Input: part model. Units: mm. Frame: model coordinates. Face numbers are marked on the shaded views. A direction names the side the tool comes from. Round coordinates to 2 decimals unless told otherwise and drop trailing zeros. Write each loop counter-clockwise with the first axis right and the second up, starting at its lowest first coordinate (ties: lowest second). Pieces come first, ordered by that corner, then holes. Notation, with made-up numbers: (9.25, -28.5) -> (34.25, -28.5) arc R8 ccw to (34.25, -19.5) -> close; hole circle Ø10 at (57.25, -26). An arc over 180 degrees is marked (long way). Use CSV: the item, a comma, the result in double quotes.
Autodesk Fusion 360 part; units mm, degrees
sketch "Sketch1" plane through (0, 0, 0) normal (0, 1, 0) x (1, 0, 0)
  line L0 (-7, -13) -> (7, -13)
  line L1 (7, -13) -> (7, 0)
  line L2 (7, 0) -> (-7, 0)
  line L3 (-7, 0) -> (-7, -13)
  line L4 (-3.5, -13) -> (3.5, -13) construction
  line L5 (3.5, -13) -> (3.5, -8.75) construction
  line L6 (3.5, -8.75) -> (-3.5, -8.75) construction
  line L7 (-3.5, -8.75) -> (-3.5, -13) construction
  line L8 (-3.5, -11.75) -> (-2.25, -13) construction
  line L9 (2.25, -13) -> (3.5, -11.75) construction
  line L10 (0, -8.75) -> (0, 0) construction
  dimension "d3" = 7
  dimension "d4" = 1.25
  dimension "d5" = 1.25
  dimension "d6" = 3
  dimension "d7" = 45
  dimension "d8" = 3.5
  dimension "d9" = 3.5
  dimension "d10" = 13
extrude "Extrude1" add sketch "Sketch1" along normal mid plane 80
sketch "Sketch2" plane through (0, 0, 0) normal (0, 0, 1) x (1, 0, 0)
  line L0 (-7, -40) -> (7, -40)
  line L1 (7, -40) -> (7, -45)
  line L2 (2, -50) -> (-2, -50)
  line L3 (-7, -45) -> (-7, -40)
  arc A0 (2, -50) -> (7, -45) centre (2, -45) ccw
  arc A1 (-7, -45) -> (-2, -50) centre (-2, -45) ccw
  line L4 (7, -40) -> (-7, -40)
  point P0 (7, -50)
  dimension "d13" = 10
  dimension "d14" = 5
extrude "Extrude2" add sketch "Sketch2" along normal blind 5
sketch "Sketch3" plane through (0, 0, 5) normal (0, 0, 1) x (-1, 0, 0)
  line L0 (7, 40) -> (7, 45)
  arc A0 (7, 45) -> (2, 50) centre (2, 45) ccw
  line L1 (2, 50) -> (-2, 50)
  arc A1 (-2, 50) -> (-7, 45) centre (-2, 45) ccw
  line L2 (-7, 45) -> (-7, 40)
  line L3 (-7, 40) -> (7, 40)
  circle A2 centre (0, 45) radius 1.75
  line L4 (-7, 45) -> (7, 45) construction
  dimension "d20" = 3.5
extrude "Extrude3" cut sketch "Sketch3" against normal blind 5 contours A2
chamfer "Chamfer1" distance 1.5 angle 60 1 edges at (1.6316, -45.6328, 5) measured on face at (-5.1922, -43.0802, 5)
mirror "Mirror1" about plane through (0, 0, 0) normal (0, 1, 0) of "Extrude2", "Extrude3", "Chamfer1"
sketch "Sketch4" plane through (0, -40, 0) normal (0, -1, 0) x (1, 0, 0)
  line L0 (-7, 5) -> (7, 5)
  line L1 (7, 5) -> (7, 13)
  line L2 (7, 13) -> (-7, 13)
  line L3 (-7, 13) -> (-7, 5)
  line L4 (-3.5, 8.75) -> (-3.5, 13) construction
  line L5 (-3.5, 11.75) -> (-2.25, 13) construction
  line L6 (2.25, 13) -> (3.5, 11.75) construction
  line L7 (3.5, 13) -> (3.5, 8.75) construction
  line L8 (3.5, 8.75) -> (-3.5, 8.75) construction
  line L9 (3.6, 13) -> (3.6, 8.65)
  line L10 (3.6, 8.65) -> (-3.6, 8.65)
  line L11 (-3.6, 8.65) -> (-3.6, 13)
  line L12 (-2.25, 13) -> (-3.6, 11.65)
  line L13 (2.25, 13) -> (3.6, 11.65)
  dimension "d25" = -0.1
extrude "Extrude4" cut sketch "Sketch4" against normal up to surface (80 mm away) contours L2 L9 L10 L11 L12 L13
sketch "Sketch5" plane through (-7, 0, 0) normal (-1, 0, 0) x (0, -1, 0)
  line L0 (40, 13) -> (-40, 13)
  line L1 (-40, 13) -> (-40, 5)
  line L2 (-40, 5) -> (-45, 5)
  line L3 (-45, 5) -> (-45, 0)
  line L4 (-45, 0) -> (45, 0)
  line L5 (45, 0) -> (45, 5)
  line L6 (45, 5) -> (40, 5)
  line L7 (40, 5) -> (40, 13)
  line L8 (-17.5, 13) -> (17.5, 13)
  line L9 (17.5, 13) -> (17.5, 5)
  line L10 (17.5, 5) -> (-17.5, 5)
  line L11 (-17.5, 5) -> (-17.5, 13)
  line L12 (0, 0) -> (0, 5) construction
  dimension "d28" = 35
extrude "Extrude5" cut sketch "Sketch5" against normal up to surface (14 mm away) contours L0 L8 L9 L10 L11
chamfer "Chamfer2" distance 0.75 angle 45 10 edges at (-2.925, -40, 12.325) (-3.6, -40, 10.15) (0, -40, 8.65) (3.6, -40, 10.15) (2.925, -40, 12.325) (2.925, 40, 12.325) (3.6, 40, 10.15) (0, 40, 8.65) (-3.6, 40, 10.15) (-2.925, 40, 12.325)
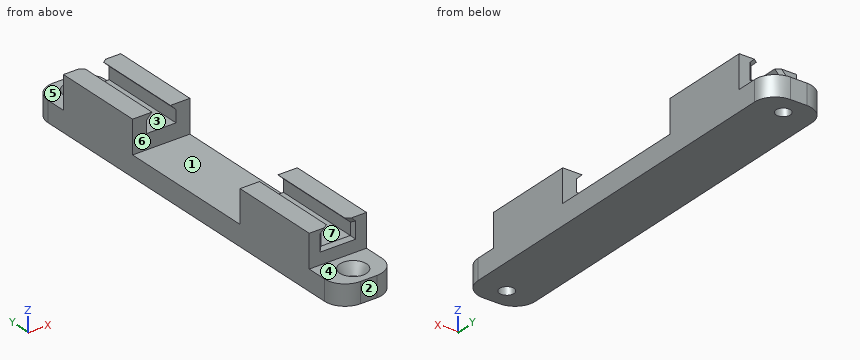
Item 1: Section query A-A on z = 10.5. Return the cut outline in (x, y).
Worked answers:
outline,"(-7, -40) -> (-4.35, -40) -> (-3.6, -39.25) -> (-3.6, -17.5) -> (-7, -17.5) -> close; (-7, 17.5) -> (-3.6, 17.5) -> (-3.6, 39.25) -> (-4.35, 40) -> (-7, 40) -> close; (3.6, -39.25) -> (4.35, -40) -> (7, -40) -> (7, -17.5) -> (3.6, -17.5) -> close; (3.6, 17.5) -> (7, 17.5) -> (7, 40) -> (4.35, 40) -> (3.6, 39.25) -> close"
Item 2: Section query D-D on z = 1.5. Return the cut outline in (x, y), plus the area to 3 significant figures.
Worked answers:
outline,"(-7, -45) arc R5 ccw to (-2, -50) -> (2, -50) arc R5 ccw to (7, -45) -> (7, 45) arc R5 ccw to (2, 50) -> (-2, 50) arc R5 ccw to (-7, 45) -> close; hole circle Ø3.5 at (0, -45); hole circle Ø3.5 at (0, 45)"
area,"1,360 mm²"
Item 3: Section query C-C on x = 0. Return the cut outline in (y, z), plus the area to 3 significant figures.
Worked answers:
outline,"(-50, 0) -> (-46.75, 0) -> (-46.75, 2.4) -> (-48.25, 5) -> (-50, 5) -> close; (-43.25, 0) -> (43.25, 0) -> (43.25, 2.4) -> (41.75, 5) -> (40, 5) -> (40, 7.9) -> (39.25, 8.65) -> (17.5, 8.65) -> (17.5, 5) -> (-17.5, 5) -> (-17.5, 8.65) -> (-39.25, 8.65) -> (-40, 7.9) -> (-40, 5) -> (-41.75, 5) -> (-43.25, 2.4) -> close; (46.75, 0) -> (50, 0) -> (50, 5) -> (48.25, 5) -> (46.75, 2.4) -> close"
area,"621 mm²"
Item 4: Pull-direction query (Y, two-part tool) for the marked faces 1, 2 and 3; classes: +Y half, -Y half, draft (parallel to the pull), parting line (faces both ways), or undercut.
Worked answers:
face 1,"undercut"
face 2,"-Y half"
face 3,"draft"
Item 5: Section query B-B on y = -33.5. Return the cut outline in (x, z), plus the area to 3 significant figures.
Worked answers:
outline,"(-7, 0) -> (7, 0) -> (7, 13) -> (2.25, 13) -> (3.6, 11.65) -> (3.6, 8.65) -> (-3.6, 8.65) -> (-3.6, 11.65) -> (-2.25, 13) -> (-7, 13) -> close"
area,"153 mm²"
Item 6: Set-up query: the marked faces 4, 5, 6 and 7. Return all of +Z, -Z, +X, -X, +Y, -Y with unobstructed straight access to the full face (end or side cutting, diameter ignored); none if empty.
Worked answers:
face 4,"+Z, +X, -X, -Y"
face 5,"+Z, +X, -X, +Y"
face 6,"+Z, +X, -X"
face 7,"+Y, -Y"
Item 7: First-contact query: pin 1 Ø6.5 at (x, z) = (1, 9) entering from -Y; pin 2 Ø1.5 at (x, y) = (2, 0) entering from +Z; pin 3 Ø2.5 at (x, z) = (1.5, 8) entering from +Y; pin 4 Ø3 at (x, y) = (0, -45) entering from +Z. Flat tips, straight axial feed; report the tip coordinate or a pass-through.
Worked answers:
pin 1,"stops at y = -40"
pin 2,"stops at z = 5"
pin 3,"stops at y = 40"
pin 4,"passes through"
Item 8: Line query: line 1 (Y direction, x = 0, z = 1.45); line 2 (X direction, y = -45, z = 1.55); line 3 (X direction, y = 39, z = 10.5). Output: solid intervals per line, ascending.
Worked answers:
line 1,"y = -50 to -46.75, -43.25 to 43.25, 46.75 to 50"
line 2,"x = -7 to -1.75, 1.75 to 7"
line 3,"x = -7 to -3.6, 3.6 to 7"
